Check sheet for the modelled part. Datum: model origin and axes. Units: mm. A direction names the side the tool comes from. Give positions to 0.01 mm unless a question says otherwise; leave off trailing zeros. Write each loop counter-clockwise with the first axis right and the second up, starting at its lowest first coordinate (ties: lowest second). Pieces come first, ordered by that corner, then holes. Notation, with made-up numbers: (51, 39.25) -> (78, 39.25) arc R26 ccw to (78, 55.25) -> close; hole circle Ø11 at (-18, 23.25). An arc over 180 degrees is marked (long way). Use a Markdown table: item, result. Add a question column.
1. Cross-section at C-C (x = -3.5). Enter the section's corners in (y, z).
2. Cross-section at D-D (y = 10.5). Enter the section's corners in (x, z).
3. Gauge pin test, flat ends, axial feed: P1, Ø4, axis at x = 12, z = 13, coming from the -Y side; P2, Ø12.5, axis at x = -3, z = -5.5, coming from the -Y side; P3, Ø5, axis at x = 12.5, z = -4.5, coming from the -Y side. Record the tip position at first contact, or that the pin passes through.
4. Release check for a two-part mould opening along Y. For faces 1 (the flat face through (0, 12, 19.05)), 2 (the cylindrical face through (-9.523, 36.894, 0.267)), 3 (the flat face through (23.93, 28.39, 0.27)) record: released by +Y, released by -Y, zero draft, split by the parting line, or undercut.
5. Cross-section at A-A (z = -3.5). Enter the section's corners in (x, y) (3 decimals), then the cut area to 3 significant figures.
6. Cross-section at B-B (y = -15). Enter the section's corners in (x, z) (3 decimals), then the cut area to 3 significant figures.
7. Scan lines: probe 1 along X at (y, z) = (-24, 10) (3 decimals); probe 2 along Y at (x, z) = (-6.5, 17.5); probe 3 along X at (y, z) = (40.5, 15.5). Record each from-to range of solid material in increasing order. Write a range as [from, to].
8. Set-up check for faces 4 (the flat face through (0, 37, 0)), 5 (the flat face through (-24, -32.746, 0)), 6 (the flat face through (-15.875, -14, 0)): record each of +Z, -Z, +X, -X, +Y, -Y from which the full face is reachable in a straight line by a thin tool's end or side.
from build123d import *

# Parameters (mm, degrees)
BOSS_EXTRUDE1_DEPTH = 19.05


with BuildPart() as part:
    # Sketch1 → Boss-Extrude1 (new, symmetric)
    with BuildSketch(Plane.XY):
        with BuildLine():
            Line((-12.7, 8.528712184), (0, 8.528712184))
            Line((0, 8.528712184), (12.7, 8.528712184))
            ThreePointArc((12.7, 8.528712184), (14.94506403, 7.598776215), (15.875, 5.353712184))
            Line((15.875, 5.353712184), (15.875, -32.746287816))
            Line((15.875, -32.746287816), (31.75, -32.746287816))
            Line((31.75, -32.746287816), (31.75, 3.774872893))
            ThreePointArc((31.75, 3.774872893), (31.301172558, 8.528712184), (29.970552126, 13.11454726))
            Line((29.970552126, 13.11454726), (17.715414094, 44.108467959))
            ThreePointArc((17.715414094, 44.108467959), (0, 56.153712184), (-17.715414094, 44.108467959))
            Line((-17.715414094, 44.108467959), (-29.970552126, 13.11454726))
            ThreePointArc((-29.970552126, 13.11454726), (-31.301172558, 8.528712184), (-31.75, 3.774872893))
            Line((-31.75, 3.774872893), (-31.75, -32.746287816))
            Line((-31.75, -32.746287816), (-15.875, -32.746287816))
            Line((-15.875, -32.746287816), (-15.875, 5.353712184))
            ThreePointArc((-15.875, 5.353712184), (-14.94506403, 7.598776215), (-12.7, 8.528712184))
        make_face()
        with BuildLine():
            Line((0, 46.628712184), (0, 27.578712184))
            ThreePointArc((0, 27.578712184), (-9.525, 37.103712184), (0, 46.628712184))
        make_face(mode=Mode.SUBTRACT)
    extrude(amount=BOSS_EXTRUDE1_DEPTH, both=True)


solid = part.part
Worked answers:
| question | item | result |
|---|---|---|
| 1 | outline | (8.53, -19.05) -> (28.25, -19.05) -> (28.25, 19.05) -> (8.53, 19.05) -> close; (45.96, -19.05) -> (55.83, -19.05) -> (55.83, 19.05) -> (45.96, 19.05) -> close |
| 2 | outline | (-30.84, -19.05) -> (30.84, -19.05) -> (30.84, 19.05) -> (-30.84, 19.05) -> close |
| 3 | P1 | stops at y = 8.25 |
| 3 | P2 | stops at y = 8.53 |
| 3 | P3 | stops at y = 7.54 |
| 4 | face 1 | zero draft |
| 4 | face 2 | undercut |
| 4 | face 3 | released by +Y |
| 5 | outline | (-31.75, -32.746) -> (-15.875, -32.746) -> (-15.875, 5.354) arc R3.175 cw to (-12.7, 8.529) -> (12.7, 8.529) arc R3.175 cw to (15.875, 5.354) -> (15.875, -32.746) -> (31.75, -32.746) -> (31.75, 3.775) arc R25.4 ccw to (29.971, 13.115) -> (17.715, 44.108) arc R19.05 ccw to (-17.715, 44.108) -> (-29.971, 13.115) arc R25.4 ccw to (-31.75, 3.775) -> close; hole (0, 27.579) -> (0, 46.629) arc R9.525 ccw to start |
| 5 | area | 3,240 mm² |
| 6 | outline | (-31.75, -19.05) -> (-15.875, -19.05) -> (-15.875, 19.05) -> (-31.75, 19.05) -> close; (15.875, -19.05) -> (31.75, -19.05) -> (31.75, 19.05) -> (15.875, 19.05) -> close |
| 6 | area | 1,210 mm² |
| 7 | probe 1 | x = [-31.75, -15.875], [15.875, 31.75] |
| 7 | probe 2 | y = [8.53, 30.14], [44.07, 55.01] |
| 7 | probe 3 | x = [-19.14, -8.9], [0, 19.14] |
| 8 | face 4 | +Z, -Z |
| 8 | face 5 | +Z, -Z, +X, -X, -Y |
| 8 | face 6 | +Z, -Z, -Y |
